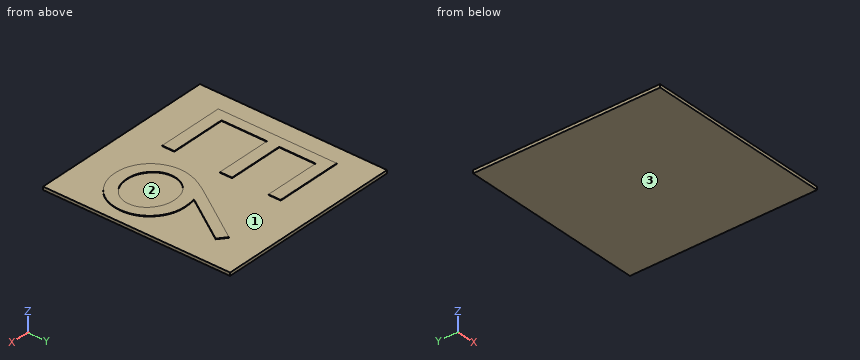
from build123d import *

# Parameters (mm, degrees)
SKETCH1_W           = 76.2
SKETCH1_H           = 76.2
BOSS_EXTRUDE1_DEPTH = 1.27
BOSS_EXTRUDE2_DEPTH = 0.254


with BuildPart() as part:
    # Sketch1 → Boss-Extrude1 (new body)
    with BuildSketch(Plane.XY):
        with Locations((38.1, 38.1)):
            Rectangle(SKETCH1_W, SKETCH1_H)
    extrude(amount=BOSS_EXTRUDE1_DEPTH)

    # Sketch2 → Boss-Extrude2 (add)
    # profile 1 of 2: a face of its own
    with BuildSketch(Plane.XY.offset(1.27)):
        Polygon((7.438286123, 61.974293726), (34.661875867, 61.974293726), (34.661875867, 57.024550136), (11.769311764, 57.024550136), (11.769311764, 42.175319367), (34.661875867, 42.175319367), (34.661875867, 37.225575777), (11.769311764, 37.225575777), (11.769311764, 18.664037315), (34.661875867, 18.664037315), (34.661875867, 13.714293726), (7.438286123, 13.714293726), align=None)
    # profile 2 of 2: a face of its own
    with BuildSketch(Plane.XY.offset(1.27)):
        with BuildLine():
            Line((61.266747661, 63.211729623), (64.602024104, 60.591845809))
            Line((64.602024104, 60.591845809), (51.850633879, 41.092562956))
            add(Edge.make_bspline(
                [(51.850633879, 41.092562956), (52.699600041, 41.227882075), (54.35560453, 41.491837316), (56.031824605, 41.535380872), (56.848714809, 41.556601418)],
                knots=[0, 0, 0, 0, 1.025318673, 2, 2, 2, 2], degree=3))
            add(Edge.make_bspline(
                [(56.848714809, 41.556601418), (57.339208715, 41.543418004), (58.304731374, 41.517466845), (59.722290309, 41.317755235), (61.084448609, 41.003029549), (62.38556044, 40.544252671), (63.630295899, 39.958205922), (64.82579808, 39.255831671), (65.949594368, 38.400861918), (67.016156628, 37.445797128), (67.984487977, 36.387979507), (68.84180696, 35.265571362), (69.561939808, 34.079742071), (70.146215653, 32.831092257), (70.599926922, 31.521546684), (70.930682279, 30.152780852), (71.126198607, 28.723850905), (71.152748374, 27.752057551), (71.166234841, 27.258416322)],
                knots=[0, 0, 0, 0, 1.04369286, 2.054478336, 3.041073146, 4.015093852, 4.984733326, 5.965804835, 6.960378782, 7.985147595, 9.009457201, 10.008161701, 10.986880575, 11.956520048, 12.937015923, 13.931873656, 14.949455224, 16, 16, 16, 16], degree=3))
            add(Edge.make_bspline(
                [(71.166234841, 27.258416322), (71.146612258, 26.583056175), (71.107999657, 25.254107236), (70.723246173, 23.318512993), (70.125378614, 21.47453265), (69.270797037, 19.751606922), (68.20931995, 18.152097205), (66.914882058, 16.734832473), (65.433389845, 15.470833616), (63.75826045, 14.413848347), (61.955501751, 13.550641706), (60.061613924, 12.930635254), (58.094989329, 12.548919759), (56.760192076, 12.501065106), (56.084984841, 12.476857828)],
                knots=[0, 0, 0, 0, 1.031375318, 2.029502543, 3.004789286, 3.987476834, 4.960371455, 5.9300674, 6.912260825, 7.929083631, 8.949397511, 9.960523116, 10.96833055, 12, 12, 12, 12], degree=3))
            add(Edge.make_bspline(
                [(56.084984841, 12.476857828), (55.43558862, 12.497929602), (54.149248406, 12.539669097), (52.257004221, 12.911490858), (50.438801587, 13.514149366), (48.70737921, 14.344418247), (47.10348413, 15.393147799), (45.668567668, 16.655660825), (44.409784514, 18.104970192), (43.362203027, 19.740851094), (42.531321197, 21.49875548), (41.908216687, 23.331768956), (41.544250201, 25.233212704), (41.493390272, 26.522184069), (41.467773302, 27.17140911)],
                knots=[0, 0, 0, 0, 1.012016664, 2.004627821, 2.994792927, 3.992885782, 4.990978636, 5.973936114, 6.964471063, 7.975201453, 8.993600317, 9.990122807, 10.98767138, 12, 12, 12, 12], degree=3))
            add(Edge.make_bspline(
                [(41.467773302, 27.17140911), (41.484063741, 27.668412421), (41.517325705, 28.683198219), (41.749571996, 30.22012793), (42.122756852, 31.792729417), (42.540691849, 33.126831527), (42.98227926, 34.219734684), (43.349779706, 35.100872529), (43.80720172, 36.007623784), (44.294950113, 36.971081405), (44.856929112, 37.9664154), (45.467978609, 39.010260853), (46.144992652, 40.086016622), (46.619597525, 40.816041439), (46.862220418, 41.189237636)],
                knots=[0, 0, 0, 0, 1.173818275, 2.396712641, 3.66331629, 4.989737886, 5.693666774, 6.447286557, 7.243889047, 8.091586357, 8.998013824, 9.943181721, 10.948533338, 12, 12, 12, 12], degree=3))
            Line((46.862220418, 41.189237636), (61.266747661, 63.211729623))
        make_face()
        with BuildLine():
            add(Edge.make_bspline(
                [(55.939972822, 36.606857828), (55.572338554, 36.596129717), (54.854242034, 36.5751746), (53.800692939, 36.453486984), (52.803596506, 36.224333811), (51.849742657, 35.932480331), (50.956964331, 35.531190713), (50.118773071, 35.043739908), (49.331927527, 34.46984332), (48.604669296, 33.817631329), (47.945304453, 33.103548337), (47.377475489, 32.338702868), (46.887672338, 31.541527599), (46.489433316, 30.705361848), (46.1793273, 29.830525256), (45.955011361, 28.921041435), (45.830173065, 27.970811602), (45.809404284, 27.32643715), (45.798798943, 26.997394687)],
                knots=[0, 0, 0, 0, 1.129588631, 2.206414736, 3.251139165, 4.268635594, 5.265702196, 6.250456724, 7.242448911, 8.251968645, 9.246821453, 10.222880186, 11.173611482, 12.116736599, 13.062300278, 14.020270554, 14.989073742, 16, 16, 16, 16], degree=3))
            add(Edge.make_bspline(
                [(45.798798943, 26.997394687), (45.807435574, 26.67129525), (45.824370719, 26.031862801), (45.978145278, 25.089563143), (46.213034728, 24.182759006), (46.562442586, 23.316125246), (46.979228193, 22.476452015), (47.529465606, 21.694153479), (48.139151915, 20.921716741), (48.867932152, 20.21847931), (49.650066294, 19.564120257), (50.485670303, 18.992166819), (51.356555921, 18.502863182), (52.27448073, 18.119387876), (53.226421418, 17.804673567), (54.220309287, 17.583208713), (55.256835574, 17.458001231), (55.958976354, 17.437205396), (56.317004072, 17.426601418)],
                knots=[0, 0, 0, 0, 0.989467248, 1.94019797, 2.891935182, 3.827694429, 4.772920941, 5.730924762, 6.725747692, 7.756678648, 8.79901574, 9.819492441, 10.826891316, 11.826466727, 12.835195252, 13.867842842, 14.912794438, 16, 16, 16, 16], degree=3))
            add(Edge.make_bspline(
                [(56.317004072, 17.426601418), (56.675031203, 17.437206228), (57.377170832, 17.458003693), (58.413705458, 17.583199356), (59.407562503, 17.804707901), (60.359615219, 18.119263413), (61.277126494, 18.503324899), (62.147250454, 18.989122741), (62.974952109, 19.567637667), (63.757599691, 20.217361058), (64.483346509, 20.925719296), (65.107655503, 21.687258269), (65.641042027, 22.482774666), (66.074474561, 23.31281757), (66.420033966, 24.18328302), (66.65611454, 25.089422761), (66.809571535, 26.031899554), (66.826550316, 26.671307663), (66.8352092, 26.997394687)],
                knots=[0, 0, 0, 0, 1.087397944, 2.132534446, 3.165364764, 4.174271784, 5.174024072, 6.181601208, 7.194203697, 8.236725232, 9.267838612, 10.269026844, 11.221737037, 12.171628256, 13.107553087, 14.05945871, 15.010357665, 16, 16, 16, 16], degree=3))
            add(Edge.make_bspline(
                [(66.8352092, 26.997394687), (66.827621446, 27.326866409), (66.812729152, 27.97351225), (66.644288672, 28.92061638), (66.41067754, 29.835146224), (66.057924094, 30.711354081), (65.599639622, 31.545782266), (65.041431273, 32.342645883), (64.395677032, 33.108054272), (63.649749243, 33.819031738), (62.837737046, 34.46912259), (61.974357575, 35.042996816), (61.0710962, 35.527320066), (60.128868754, 35.931423139), (59.136879177, 36.223044174), (58.111142672, 36.452668606), (57.038540143, 36.57486317), (56.31082611, 36.596057103), (55.939972822, 36.606857828)],
                knots=[0, 0, 0, 0, 0.978206639, 1.919901502, 2.851605144, 3.780102724, 4.718870031, 5.675451981, 6.667674623, 7.690630536, 8.733308323, 9.756129687, 10.767539656, 11.776269907, 12.797430371, 13.836405707, 14.897401972, 16, 16, 16, 16], degree=3))
        make_face(mode=Mode.SUBTRACT)
    extrude(amount=BOSS_EXTRUDE2_DEPTH)


solid = part.part
Geometry: final body of the model. Coordinates: model frame, mm. Face numbers are marked on the shaded views. Give positions to 0.01 mm unless a question says otherwise; leave off trailing zeros. Order: outer loops, then holes, each group sorted by start corner. A loop starts at its lowest first (then second) coordinate and runs counter-clockwise, first axis right, second up. Notation, with made-up numbers: (80.5, -17.75) - (117.5, -17.75) arc R23 ccw to (117.5, 7.25) - close; hole circle Ø3 at (-21.5, 38.25). An arc over 180 degrees is marked (long way). Use CSV: the item, a comma, the result in double quotes.
1. Section query A-A (x = 20). Output: boundary loops of the cut face in (y, z), plus the area to 3 significant figures.
Answers below:
outline,"(0, 0) - (76.2, 0) - (76.2, 1.27) - (61.97, 1.27) - (61.97, 1.52) - (57.02, 1.52) - (57.02, 1.27) - (42.18, 1.27) - (42.18, 1.52) - (37.23, 1.52) - (37.23, 1.27) - (18.66, 1.27) - (18.66, 1.52) - (13.71, 1.52) - (13.71, 1.27) - (0, 1.27) - close"
area,"101 mm2"
2. Mould query, pull axis X, two halves, no side actions, for the marked faces 1, 2 and 3. Classes: +X half, -X half, draft (parallel to the pull), parting line (faces both ways), or undercut.
Answers below:
face 1,"undercut"
face 2,"undercut"
face 3,"draft"
3. Material intervals for line 1 along Y through (x, z) = (52, 1.45); line 2 along Z through (x, y) = (32.5, 44); line 3 along Y through (x, z) = (55, 1.45), sorted ascending. Write a range as from..to.
Answers below:
line 1,"13.02..18.24, 35.97..41.12, 41.32..49.04"
line 2,"0..1.27"
line 3,"12.52..17.5, 36.57..41.49, 45.91..53.63"
4. Section query B-B (y = 11.5). Output: boundary loops of the cut face in (x, z), plus the area to 3 significant figures.
Answers below:
outline,"(0, 0) - (76.2, 0) - (76.2, 1.27) - (0, 1.27) - close"
area,"96.8 mm2"
